Build history of the part. All positions in model axes, mm. Round coordinates to 2 decimals unless told otherwise and drop trailing zeros. Write each loop counter-clockwise with the first axis right and the second up, starting at its lowest first coordinate (ties: lowest second). Pieces come first, ordered by that corner, then holes. Notation, with made-up numbers: M 24,-36 L 47,-36 A25 cw 47,-18 Z; hole C -1.5,36.25 d1. An arc over 180 degrees is marked long. Use a Markdown table: item, result.
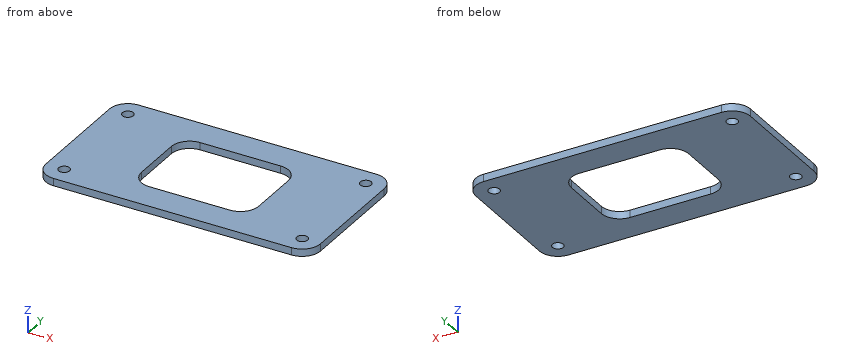
from build123d import *

# Parameters (mm, degrees)
SKETCH1_R           = 1.5
BOSS_EXTRUDE1_DEPTH = 2


with BuildPart() as part:
    # Sketch1 → Boss-Extrude1 (new body)
    with BuildSketch(Plane.XY):
        with BuildLine():
            Line((32.5, 20), (-32.5, 20))
            ThreePointArc((-32.5, 20), (-36.035533906, 18.535533906), (-37.5, 15))
            Line((-37.5, 15), (-37.5, -15))
            ThreePointArc((-37.5, -15), (-36.035533906, -18.535533906), (-32.5, -20))
            Line((-32.5, -20), (32.5, -20))
            ThreePointArc((32.5, -20), (36.035533906, -18.535533906), (37.5, -15))
            Line((37.5, -15), (37.5, 15))
            ThreePointArc((37.5, 15), (36.035533906, 18.535533906), (32.5, 20))
        make_face()
        with Locations((-32.5, -15)):
            Circle(SKETCH1_R, mode=Mode.SUBTRACT)
        with Locations((-32.5, 15)):
            Circle(SKETCH1_R, mode=Mode.SUBTRACT)
        with Locations((32.5, 15)):
            Circle(SKETCH1_R, mode=Mode.SUBTRACT)
        with Locations((32.5, -15)):
            Circle(SKETCH1_R, mode=Mode.SUBTRACT)
        with BuildLine():
            Line((-11, 12), (11, 12))
            ThreePointArc((11, 12), (14.535533906, 10.535533906), (16, 7))
            Line((16, 7), (16, -7))
            ThreePointArc((16, -7), (14.535533906, -10.535533906), (11, -12))
            Line((11, -12), (-11, -12))
            ThreePointArc((-11, -12), (-14.535533906, -10.535533906), (-16, -7))
            Line((-16, -7), (-16, 7))
            ThreePointArc((-16, 7), (-14.535533906, 10.535533906), (-11, 12))
        make_face(mode=Mode.SUBTRACT)
    extrude(amount=BOSS_EXTRUDE1_DEPTH)


solid = part.part
Q1. Cut at A-A on z = 1.5. Give the cut face in (x, y).
Response values:
| item | result |
|---|---|
| outline | M -37.5,-15 A5 ccw -32.5,-20 L 32.5,-20 A5 ccw 37.5,-15 L 37.5,15 A5 ccw 32.5,20 L -32.5,20 A5 ccw -37.5,15 Z; hole C -32.5,-15 d3; hole C -32.5,15 d3; hole M -16,-7 A5 ccw -11,-12 L 11,-12 A5 ccw 16,-7 L 16,7 A5 ccw 11,12 L -11,12 A5 ccw -16,7 Z; hole C 32.5,-15 d3; hole C 32.5,15 d3 |
Q2. Drill centre lines: L1, parallel to Y at x = -32.5, z = 1.4; L2, parallel to Y at x = -5.5, z = 1.2; L3, parallel to X at y = -7, z = 0.2. Where is each one in solid material? Low to high.
Response values:
| item | result |
|---|---|
| L1 | y = -20 to -16.5, -13.5 to 13.5, 16.5 to 20 |
| L2 | y = -20 to -12, 12 to 20 |
| L3 | x = -37.5 to -16, 16 to 37.5 |
Q3. Cut at B-B on x = -8. Give the cut face in (y, z), and give its area (3 significant figures).
Response values:
| item | result |
|---|---|
| outline | M -20,0 L -12,0 L -12,2 L -20,2 Z; M 12,0 L 20,0 L 20,2 L 12,2 Z |
| area | 32.0 mm2 |
Q4. Cut at C-C on y = 2.5. Give the cut face in (x, z).
Response values:
| item | result |
|---|---|
| outline | M -37.5,0 L -16,0 L -16,2 L -37.5,2 Z; M 16,0 L 37.5,0 L 37.5,2 L 16,2 Z |
